from build123d import *

# Parameters (mm, degrees)
SKETCH_1_R          = 10
EXTRUDE_1_DEPTH     = 2.5
SKETCH_3_R          = 1.6
CUT_EXTRUDE_1_DEPTH = 3.5
SKETCH_4_R          = 4.5
EXTRUDE_2_DEPTH     = 2
SKETCH_5_R          = 2.95
CUT_EXTRUDE_2_DEPTH = 2


with BuildPart() as part:
    # 草图1 → 凸台-拉伸1 (new body)
    with BuildSketch(Plane(origin=(0, 0, 0), x_dir=(1, 0, 0), z_dir=(0, 1, 0))):
        Circle(SKETCH_1_R)
    extrude(amount=EXTRUDE_1_DEPTH)

    # 草图3 → 切除-拉伸1 (cut, through all)
    with BuildSketch(Plane(origin=(0, 2.5, 0), x_dir=(1, 0, 0), z_dir=(0, 1, 0))):
        with Locations((-4.795236977, 5.099578643)):
            Circle(SKETCH_3_R)
        with Locations((-5.099578643, -4.795236977)):
            Circle(SKETCH_3_R)
        with Locations((4.795236977, -5.099578643)):
            Circle(SKETCH_3_R)
        with Locations((5.099578643, 4.795236977)):
            Circle(SKETCH_3_R)
        Circle(SKETCH_3_R)
    extrude(amount=-CUT_EXTRUDE_1_DEPTH, mode=Mode.SUBTRACT)

    # 草图4 → 凸台-拉伸2 (add)
    with BuildSketch(Plane(origin=(0, 2.5, 0), x_dir=(1, 0, 0), z_dir=(0, 1, 0))):
        Circle(SKETCH_4_R)
    extrude(amount=EXTRUDE_2_DEPTH)

    # 草图5 → 切除-拉伸2 (cut)
    with BuildSketch(Plane(origin=(0, 4.5, 0), x_dir=(1, 0, 0), z_dir=(0, 1, 0))):
        Circle(SKETCH_5_R)
    extrude(amount=-CUT_EXTRUDE_2_DEPTH, mode=Mode.SUBTRACT)


solid = part.part
Source: CAD feature listing. Evaluate the final solid. Frame: model axes, mm. A direction names the side the tool comes from. Give positions to 0.01 mm unless a question says otherwise; leave off trailing zeros. Write each loop counter-clockwise with the first axis right and the second up, starting at its lowest first coordinate (ties: lowest second). Pieces come first, ordered by that corner, then holes. Notation, with made-up numbers: M -21.75,-18.75 L 6.25,-18.75 A26 cw 6.25,0.25 Z; hole C 85.25,41 d11. An arc over 180 degrees is marked long. Return JSON: item names as keys, results as strings. Group by question number.
1) Cut plane B-B, the plane x = 0. Output: boundary loops of the cut face in (y, z).
2) Cut plane A-A, the plane z = 0. Output: boundary loops of the cut face in (x, y), then the cut area to 3 significant figures.
3) Draft query along X for faces 3 (the face through (-6.065, 1.268, -4.126)), 4 (the face through (-5, 2.5, 0)), 5 (the face through (-0.59, 3.49, -4.46)). Return one class per face: released by +X, released by -X, zero draft, split by the parting line, or undercut.
4) Cut plane C-C, the plane x = -4.75. Output: boundary loops of the cut face in (y, z), then the cut area to 3 significant figures.
5) Ray query, L1, parallel to X at y = 0.65, z = 5.5; L2, parallel to Z at x = 0, y = 3.15. Return the intervals inside material, ascending.
6) Set-up query: faces 1 (the face through (1.3, 2.5, 1.3)), 2 (the face through (-5.31, 1.27, 3.21)). Return all of +Z, -Z, +X, -X, +Y, -Y with unobstructed straight access to the full face (end or side cutting, diameter ignored); none if empty.
7) First-contact query: pin 1 Ø1.9 at (x, z) = (0, 0) entering from +Y; pin 2 Ø1.5 at (x, y) = (-1.5, 2) entering from -Z; pin 3 Ø10 at (x, z) = (-6, 7.5) entering from +Y. Flat tips, straight axial feed; report the tip coordinate or a pass-through.
8) Cut plane D-D, the plane y = 1.05. Output: boundary loops of the cut face in (x, z).
Data:
{
 "1": {"outline": "M 0,-10 L 2.5,-10 L 2.5,-4.5 L 4.5,-4.5 L 4.5,-2.95 L 2.5,-2.95 L 2.5,-1.6 L 0,-1.6 Z; M 0,1.6 L 2.5,1.6 L 2.5,2.95 L 4.5,2.95 L 4.5,4.5 L 2.5,4.5 L 2.5,10 L 0,10 Z"},
 "2": {"outline": "M -10,0 L -1.6,0 L -1.6,2.5 L -2.95,2.5 L -2.95,4.5 L -4.5,4.5 L -4.5,2.5 L -10,2.5 Z; M 1.6,0 L 10,0 L 10,2.5 L 4.5,2.5 L 4.5,4.5 L 2.95,4.5 L 2.95,2.5 L 1.6,2.5 Z", "area": "48.2 mm²"},
 "3": {"face 3": "undercut", "face 4": "zero draft", "face 5": "split by the parting line"},
 "4": {"outline": "M 0,-8.8 L 2.5,-8.8 L 2.5,-6.7 L 0,-6.7 Z; M 0,-3.5 L 2.5,-3.5 L 2.5,3.23 L 0,3.23 Z; M 0,6.36 L 2.5,6.36 L 2.5,8.8 L 0,8.8 Z", "area": "28.2 mm²"},
 "5": {"L1": "x = -8.35 to -6.54, -3.66 to 3.25, 6.34 to 8.35", "L2": "z = -4.5 to -2.95, 2.95 to 4.5"},
 "6": {"face 1": "+Y", "face 2": "+Y, -Y"},
 "7": {"pin 1": "passes through", "pin 2": "stops at z = -9.97", "pin 3": "stops at y = 2.5"},
 "8": {"outline": "C 0,0 d20; hole C -5.1,4.8 d3.2; hole C -4.8,-5.1 d3.2; hole C 0,0 d3.2; hole C 4.8,5.1 d3.2; hole C 5.1,-4.8 d3.2"}
}
